```python
from build123d import *

# Parameters (mm, degrees)
BOSS_EXTRU_1_DEPTH                                = 5
ESQUISSE2_R                                       = 13
ENL_V_MAT_EXTRU_1_DEPTH                           = 10
CHANFREIN1_SIZE                                   = 3
CHANFREIN2_SIZE                                   = 1
CHAMBRAGE_POUR_VIS_SIX_PANS_CREUX_M31_D           = 3.4
CHAMBRAGE_POUR_VIS_SIX_PANS_CREUX_M31_CBORE_D     = 6.5
CHAMBRAGE_POUR_VIS_SIX_PANS_CREUX_M31_CBORE_DEPTH = 3.4


with BuildPart() as part:
    # Esquisse1 → Boss.-Extru.1 (new, symmetric)
    with BuildSketch(Plane.XY):
        Polygon((8, 0), (20, 0), (20, -8), (0, -8), (0, 0), (0, 30), (0, 51), (6, 51), (6, 30), (8, 30), align=None)
    extrude(amount=BOSS_EXTRU_1_DEPTH, both=True)

    # Esquisse2 → Enlèv. mat.-Extru.1 (cut)
    with BuildSketch(Plane.XZ.offset(8)):
        with Locations((30, 0)):
            Circle(ESQUISSE2_R)
    extrude(amount=-ENL_V_MAT_EXTRU_1_DEPTH, mode=Mode.SUBTRACT)

    # Chanfrein1
    chanfrein1_edges = [part.edges().sort_by_distance(p)[0] for p in [
        (0, -8, 0),
    ]]
    chamfer(chanfrein1_edges, length=CHANFREIN1_SIZE)

    # Chanfrein2
    chanfrein2_edges = [part.edges().sort_by_distance(p)[0] for p in [
        (17, 0, 0),
    ]]
    chamfer(chanfrein2_edges, length=CHANFREIN2_SIZE)

    # Chambrage pour vis à six pans creux M31 (through all)
    with Locations(Plane.ZY):
        with Locations((0, 40), (0, 33)):
            CounterBoreHole(CHAMBRAGE_POUR_VIS_SIX_PANS_CREUX_M31_D / 2, CHAMBRAGE_POUR_VIS_SIX_PANS_CREUX_M31_CBORE_D / 2, CHAMBRAGE_POUR_VIS_SIX_PANS_CREUX_M31_CBORE_DEPTH)


solid = part.part
```
Check sheet for the modelled part. Datum: model origin and axes. Units: mm. A direction names the side the tool comes from. Give positions to 0.01 mm unless a question says otherwise; leave off trailing zeros. Order: outer loops, then holes, each group sorted by start corner. A loop starts at its lowest first (then second) coordinate and runs counter-clockwise, first axis right, second up. Notation, with made-up numbers: M 53.5,68 L 108.5,68 A18 ccw 108.5,82 Z; hole C -3,22.5 d11. An arc over 180 degrees is marked long. Answer in a Markdown table with one row per item.
1) Thickness scan on L1, parallel to Y at x = 4.7, z = 0; L2, parallel to Y at x = 2.75, z = 0; L3, parallel to X at y = 28, z = 1.25. Record the ranges inside material, lowest first. Write a range as [from, to].
Filled sheet:
| item | result |
|---|---|
| L1 | y = [-8, 31.3], [34.7, 38.3], [41.7, 51] |
| L2 | y = [-7.75, 29.75], [36.25, 36.75], [43.25, 51] |
| L3 | x = [0, 8] |
2) Cross-section at A-A, the plane x = 4.75. Enter the section's corners in (y, z), plus the area to 3 significant figures.
Filled sheet:
| item | result |
|---|---|
| outline | M -8,-5 L 51,-5 L 51,5 L -8,5 Z; hole C 33,0 d3.4; hole C 40,0 d3.4 |
| area | 572 mm2 |
3) Cross-section at B-B, the plane z = 0. Enter the section's corners in (x, y), plus the area to 3 significant figures.
Filled sheet:
| item | result |
|---|---|
| outline | M 0,-5 L 3,-8 L 17,-8 L 17,-1 L 16,0 L 8,0 L 8,30 L 6,30 L 6,31.3 L 3.4,31.3 L 3.4,29.75 L 0,29.75 Z; M 0,36.25 L 3.4,36.25 L 3.4,34.7 L 6,34.7 L 6,38.3 L 3.4,38.3 L 3.4,36.75 L 0,36.75 Z; M 0,43.25 L 3.4,43.25 L 3.4,41.7 L 6,41.7 L 6,51 L 0,51 Z |
| area | 435 mm2 |
4) Access from +Z, -Z, +X, -X, +Y, -Y to the whole of each face (thin tool, end or side, straight path). Record for faces 1 (the cylindrical face through (1.676, 29.827, -0.705)), 2 (the flat face through (2, -7, 0)), 3 (the flat face through (6, 43, 0)).
Filled sheet:
| item | result |
|---|---|
| face 1 | -X |
| face 2 | +Z, -Z, -X, -Y |
| face 3 | +Z, -Z, +X, +Y |
5) Gauge pin test, flat ends, axial feed: P1, Ø2.5, axis at y = 40, z = 0, coming from the +X side; P2, Ø5, axis at y = 37, z = 0, coming from the +X side; P3, Ø4.5, axis at x = 13, z = 1, coming from the +Y side; P4, Ø3, axis at y = 34.5, z = 0.5, coming from the -X side. Record the tip position at first contact, or that the pin passes through.
Filled sheet:
| item | result |
|---|---|
| P1 | passes through |
| P2 | stops at x = 6 |
| P3 | stops at y = 0 |
| P4 | stops at x = 3.4 |
6) Cross-section at C-C, the plane y = 33. Enter the section's corners in (x, z), plus the area to 3 significant figures.
Filled sheet:
| item | result |
|---|---|
| outline | M 0,-5 L 6,-5 L 6,-1.7 L 3.4,-1.7 L 3.4,-3.25 L 0,-3.25 Z; M 0,3.25 L 3.4,3.25 L 3.4,1.7 L 6,1.7 L 6,5 L 0,5 Z |
| area | 29.1 mm2 |
7) Cross-section at D-D, the plane x = 11.25. Enter the section's corners in (y, z), plus the area to 3 significant figures.
Filled sheet:
| item | result |
|---|---|
| outline | M -8,-5 L 0,-5 L 0,5 L -8,5 Z |
| area | 80.0 mm2 |
